```python
from build123d import *

# Parameters (mm, degrees)
OVERALL_DIMENSIONS_W    = 65
OVERALL_DIMENSIONS_H    = 50
RECTANGULAR_PLATE_DEPTH = 3.175
EXTERNAL_4_FILLETS_R    = 6
HOLE_POSITIONS_R        = 1
CORNER_HOLES_DEPTH      = 42.125790266
RJ45_GEOMETRY_W         = 18.55
RJ45_GEOMETRY_H         = 16.24
RJ45_CUTOUTS_DEPTH      = 42.125790266
CLIP_SLOT_GEOMETRY_W    = 6.35
CLIP_SLOT_GEOMETRY_H    = 6.2
CLIP_SLOTS_DEPTH        = 42.125790266
FILLET1_R               = 1


with BuildPart() as part:
    # overall dimensions → Rectangular Plate (new body)
    with BuildSketch(Plane.XY):
        Rectangle(OVERALL_DIMENSIONS_W, OVERALL_DIMENSIONS_H)
    extrude(amount=-RECTANGULAR_PLATE_DEPTH)

    # External 4 Fillets
    external_4_fillets_edges = [part.edges().sort_by_distance(p)[0] for p in [
        (32.5, -25, -1.5875),
        (-32.5, -25, -1.5875),
        (-32.5, 25, -1.5875),
        (32.5, 25, -1.5875),
    ]]
    fillet(external_4_fillets_edges, radius=EXTERNAL_4_FILLETS_R)

    # hole positions → Corner Holes (cut, through all)
    with BuildSketch(Plane.XY):
        with Locations((-26.5, 19)):
            Circle(HOLE_POSITIONS_R)
        with Locations(Location((26.5, 19, 0), (0, 0, 180))):
            Circle(HOLE_POSITIONS_R)
        with Locations((26.5, -19)):
            Circle(HOLE_POSITIONS_R)
        with Locations(Location((-26.5, -19, 0), (0, 0, 180))):
            Circle(HOLE_POSITIONS_R)
    extrude(amount=-CORNER_HOLES_DEPTH, mode=Mode.SUBTRACT)

    # RJ45 geometry → RJ45 cutouts (cut, through all)
    with BuildSketch(Plane.XY):
        with Locations((-23.225, 0)):
            Rectangle(RJ45_GEOMETRY_W, RJ45_GEOMETRY_H)
        with Locations((23.225, 0)):
            Rectangle(RJ45_GEOMETRY_W, RJ45_GEOMETRY_H)
    extrude(amount=-RJ45_CUTOUTS_DEPTH, mode=Mode.SUBTRACT)

    # clip slot geometry → clip slots (cut, through all)
    with BuildSketch(Plane.XY):
        with Locations((10.205, 21.9)):
            Rectangle(CLIP_SLOT_GEOMETRY_W, CLIP_SLOT_GEOMETRY_H)
        with Locations((-10.205, 21.9)):
            Rectangle(CLIP_SLOT_GEOMETRY_W, CLIP_SLOT_GEOMETRY_H)
        with Locations((-10.205, -21.9)):
            Rectangle(CLIP_SLOT_GEOMETRY_W, CLIP_SLOT_GEOMETRY_H)
        with Locations((10.205, -21.9)):
            Rectangle(CLIP_SLOT_GEOMETRY_W, CLIP_SLOT_GEOMETRY_H)
    extrude(amount=-CLIP_SLOTS_DEPTH, mode=Mode.SUBTRACT)

    # Fillet1
    fillet1_edges = [part.edges().sort_by_distance(p)[0] for p in [
        (32.5, -8.12, -1.5875),
        (13.95, -8.12, -1.5875),
        (13.95, 8.12, -1.5875),
        (32.5, 8.12, -1.5875),
        (-13.95, 8.12, -1.5875),
        (-13.95, -8.12, -1.5875),
        (-32.5, -8.12, -1.5875),
        (-32.5, 8.12, -1.5875),
    ]]
    fillet(fillet1_edges, radius=FILLET1_R)


solid = part.part
```
Build history of the part. All positions in model axes, mm. A direction names the side the tool comes from. Coordinates: 2 decimals unless noted, no trailing zeros. Order: outer loops, then holes, each group sorted by start corner. A loop starts at its lowest first (then second) coordinate and runs counter-clockwise, first axis right, second up. Notation, with made-up numbers: (-29, 7) -> (-20, 7) arc R34 cw to (-20, 38) -> close; hole circle Ø6 at (0.25, 10.5). An arc over 180 degrees is marked (long way). Answer in a Markdown table with one row per item. Add a question column.
Q1. Drop flat-ended pins along their axis: pin 1 (1 mm diameter, centred on y = -22.5, z = -2, fed in from +X); pin 2 (1.6 mm diameter, centred on y = 23, z = -1, fed in from -X); pin 3 (1 mm diameter, centred on y = 2, z = -2, fed in from +X). Give the stop position or say it passes through.
Q2. Band-saw the part on B-B, the plane z = -1. Give the number of separate pieces and of enclosed holes in the cut face, then the cut area to 3 significant figures.
Q3. Which spindle directions (+Z, -Z, +X, -X, +Y, -Y) get a long thin tool onto all of the face, cutting with end or side? Do faces 4 (the face through (-7.03, -22, -2)), 5 (the face through (20, -25, -2)), 6 (the face through (7.03, 22, -2)). Say none if no direction does.
Q4. Wall check: line 1 along Y through (x, z) = (-26.5, -0.95); line 2 along X through (y, z) = (22, -0.9); line 3 along X through (y, z) = (-19.5, -2.9). Give the ranges that are in metal, low to high. Write a range as [from, to].
Q5. Band-saw the part on A-A, the plane x = -20. List the corners of the cut face in (y, z) (3 decimals), then the cut area to 3 significant figures.
Q6. Band-saw the part on D-D, the plane x = -12. List the corners of the cut face in (y, z) (3 decimals), then the cut area to 3 significant figures.
Q7. Mould opens along X. For faces 1 (the face through (-23, 8.12, -2)), 2 (the face through (32.5, -14, -2)), 3 (the face through (10, 18.8, -2)) say: +X half, -X half, draft (parallel to the pull), parting line (faces both ways), or undercut.
Q8. Band-saw the part on C-C, the plane y = 3. List the corners of the cut face in (x, z) (3 decimals), then the cut area to 3 significant figures.
Answers follow:
| question | item | result |
|---|---|---|
| 1 | pin 1 | x = 31.7 |
| 1 | pin 2 | x = -31.58 |
| 1 | pin 3 | x = 13.95 |
| 2 | separate pieces | 1 |
| 2 | enclosed holes | 4 |
| 2 | area | 2,450 mm^2 |
| 3 | face 4 | +Z, -Z, -Y |
| 3 | face 5 | +Z, -Z, +X, -X, -Y |
| 3 | face 6 | +Z, -Z, +Y |
| 4 | line 1 | [-25, -20], [-18, -8.12], [8.12, 18], [20, 25] |
| 4 | line 2 | [-31.7, -13.38], [-7.03, 7.03], [13.38, 31.7] |
| 4 | line 3 | [-32.48, -27.37], [-25.63, -13.38], [-7.03, 7.03], [13.38, 25.63], [27.37, 32.48] |
| 5 | outline | (-25, -3.175) -> (-8.12, -3.175) -> (-8.12, 0) -> (-25, 0) -> close; (8.12, -3.175) -> (25, -3.175) -> (25, 0) -> (8.12, 0) -> close |
| 5 | area | 107 mm^2 |
| 6 | outline | (-18.8, -3.175) -> (18.8, -3.175) -> (18.8, 0) -> (-18.8, 0) -> close |
| 6 | area | 119 mm^2 |
| 7 | face 1 | draft |
| 7 | face 2 | +X half |
| 7 | face 3 | undercut |
| 8 | outline | (-13.95, -3.175) -> (13.95, -3.175) -> (13.95, 0) -> (-13.95, 0) -> close |
| 8 | area | 88.6 mm^2 |
